Input: dimensioned drawing with shaded views. Units: mm. Origin: part minimum x, y, z. A direction names the side the tool comes from. Give positions to 0.01 mm unless a question says otherwise; leave off trailing zeros. Write each loop counter-clockwise with the first axis right and the second up, starting at its lowest first coordinate (ties: lowest second). Pieces come first, ordered by that corner, then holes. Notation, with made-up numbers: (71.25, 72) -> (108.25, 72) arc R19 ccw to (108.25, 79) -> close; hole circle Ø8 at (-37.5, 76). An arc over 180 degrees is marked (long way). Answer as a JSON object with one key per item and string values. Group by question number.
(1) Material intervals for probe 1 along Z at (x, y) = (25.5, 6.5); probe 2 along Y at (x, z) = (15.24, 5.5); probe 3 along Y at (x, z) = (15, 2), sorted ascending.
(2) Section query A-A on y = 15.24. Output: boundary loops of the cut face in (x, z), plus the area to 3 significant figures.
(3) Draft query along Z for the marked faces 1, 2 and 3. Return one class per face: +Z half, -Z half, draft (parallel to the pull), parting line (faces both ways), or undercut.
(4) Set-up query: the marked faces 4 and 5. Return all of +Z, -Z, +X, -X, +Y, -Y with unobstructed straight access to the full face (end or side cutting, diameter ignored); none if empty.
(5) Section query D-D on y = 5. Output: boundary loops of the cut face in (x, z).
(6) Section query C-C on z = 8.5. Output: boundary loops of the cut face in (x, y).
(7) Contact query for flat-ended pins moving along their axis: pin 1 Ø1.5 at (y, z) = (17, 6.5) entering from +X; pin 2 Ø4 at (y, z) = (21.5, 7) entering from +X; pin 3 Ø1.5 at (x, z) = (17, 7) entering from -Y. Output: stop coordinate, or through.
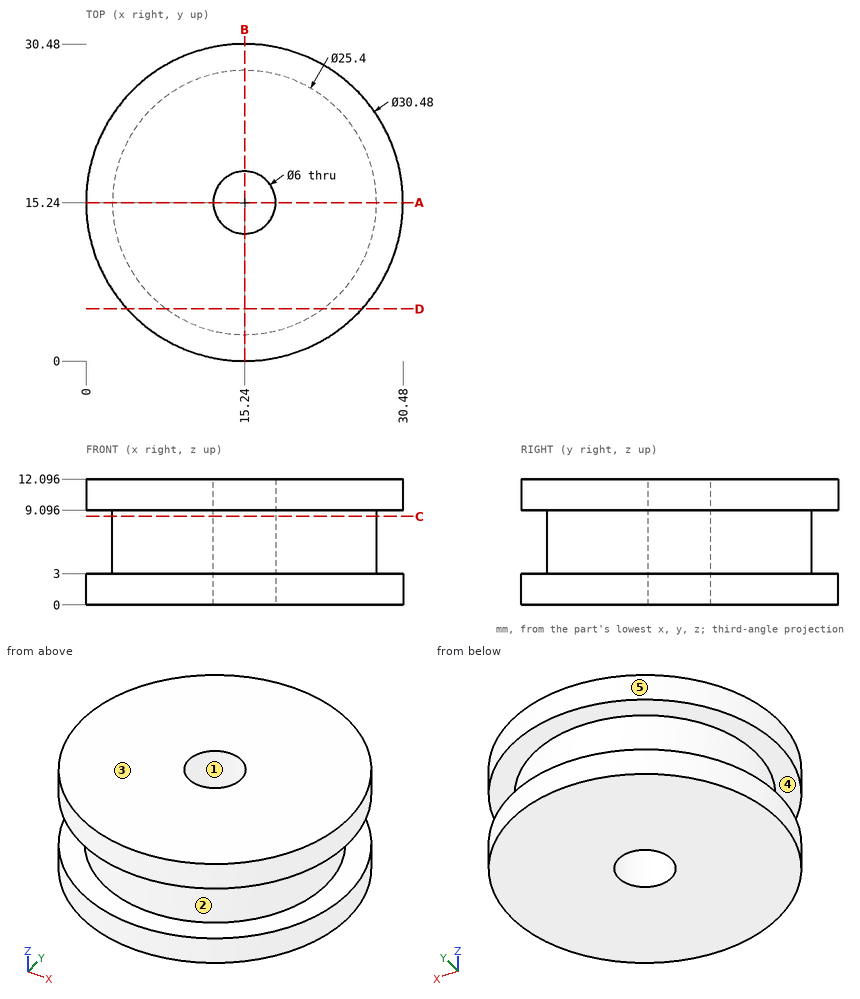
Answer list:
{
 "1": {"probe 1": "0 to 3, 9.1 to 12.1", "probe 2": "2.54 to 12.24, 18.24 to 27.94", "probe 3": "0 to 12.25, 18.23 to 30.48"},
 "2": {"outline": "(0, 0) -> (12.24, 0) -> (12.24, 12.1) -> (0, 12.1) -> (0, 9.1) -> (2.54, 9.1) -> (2.54, 3) -> (0, 3) -> close; (18.24, 0) -> (30.48, 0) -> (30.48, 3) -> (27.94, 3) -> (27.94, 9.1) -> (30.48, 9.1) -> (30.48, 12.1) -> (18.24, 12.1) -> close", "area": "265 mm2"},
 "3": {"face 1": "draft", "face 2": "undercut", "face 3": "+Z half"},
 "4": {"face 4": "none", "face 5": "+Z, -Z"},
 "5": {"outline": "(3.95, 0) -> (26.53, 0) -> (26.53, 3) -> (22.75, 3) -> (22.75, 9.1) -> (26.53, 9.1) -> (26.53, 12.1) -> (3.95, 12.1) -> (3.95, 9.1) -> (7.73, 9.1) -> (7.73, 3) -> (3.95, 3) -> close"},
 "6": {"outline": "circle Ø25.4 at (15.24, 15.24); hole circle Ø6 at (15.24, 15.24)"},
 "7": {"pin 1": "x = 27.9", "pin 2": "x = 27.2", "pin 3": "y = 2.58"}
}
